Could you check a few things on this model? Use its own coordinates, in mm. A direction names the side the tool comes from. Coordinates: 2 decimals unless noted, no trailing zeros. Write each loop counter-clockwise with the first axis right and the second up, starting at its lowest first coordinate (ties: lowest second). Pieces come first, ordered by that corner, then holes. Notation, with made-up numbers: (20, -23) - (73, -23) arc R19 cw to (73, 2) - close; hole circle Ø3 at (-33, -13.5). An arc over 180 degrees is marked (long way). Answer as a JSON object with one key per item and string values. Group by question number.
1) Please list where these lines run through material, in increasing order: line 1 along Z through (x, y) = (49.5, 8.75) (3 decimals); line 2 along Y through (x, z) = (72, -6) (3 decimals); line 3 along X through (y, z) = (22.5, -28.5).
2) If we section it at B-B (x = 40): Write out the boundary of the cut face in (y, z) (3 decimals), plus the area to 3 significant figures.
3) If we section it at D-D (z = -9): Write out the boundary of the cut face in (x, y) (3 decimals), plus the area to 3 significant figures.
4) If we section it at C-C (y = 17.25): Write out the boundary of the cut face in (x, z) (3 decimals), plus the area to 3 significant figures.
5) We'd pull the mould along Z, two halves only. Please class faces 4 (the flat face through (0, 23, -25)), 5 (the flat face through (26, 24, -38.1)), 6 (the flat face through (50, 13, -50.8)), 7 (the flat face through (50, 22.225, -26)): released by +Z, released by -Z, zero draft, split by the parting line, or undercut.
6) If we section it at A-A (z = -27): Write out the boundary of the cut face in (x, y) (3 decimals).
7) On a 3-axis mill with a long thin cutter (end or side, diameter ignored), from which of +Z, -Z, +X, -X, +Y, -Y can I reach the whole of each face in a straight line? I mean faces 1 (the flat face through (50, 13, 0)), 2 (the flat face through (25, 24, -12.7)), 3 (the flat face through (50, 3.175, -25)). Say none if no direction works.
Autodesk Fusion 360 part; units mm, degrees
sketch "Sketch1" plane through (0, 0, 0) normal (1, 0, 0) x (0, 0, -1)
  line L0 (0, 0) -> (50.8, 0)
  line L1 (50.8, 0) -> (50.8, 25.4)
  line L2 (50.8, 25.4) -> (0, 25.4)
  line L3 (0, 25.4) -> (0, 0)
  line L4 (3.175, 3.175) -> (47.625, 3.175)
  line L5 (47.625, 3.175) -> (47.625, 22.225)
  line L6 (47.625, 22.225) -> (3.175, 22.225)
  line L7 (3.175, 22.225) -> (3.175, 3.175)
  dimension "d1" = 50.8
  dimension "d2" = 25.4
  dimension "d3" = -3.175
extrude "Extrude1" add sketch "Sketch1" along normal blind 101.6
sketch "Sketch2" plane through (0, 25.4, 0) normal (0, 1, 0) x (-1, 0, 0)
  line L0 (0, -50.8) -> (0, 0)
  line L1 (0, 0) -> (-101.6, 0)
  line L2 (-101.6, 0) -> (-101.6, -50.8)
  line L3 (-101.6, -50.8) -> (0, -50.8)
  line L4 (-12.7, -12.7) -> (-38.1, -12.7)
  line L5 (-38.1, -12.7) -> (-38.1, -38.1)
  line L6 (-38.1, -38.1) -> (-12.7, -38.1)
  line L7 (-12.7, -38.1) -> (-12.7, -12.7)
  dimension "d6" = 25.4
  dimension "d7" = 25.4
  dimension "d8" = 12.7
  dimension "d11" = 12.7
extrude "Extrude2" cut sketch "Sketch2" against normal blind 3.175 contours L4 L5 L6 L7
Here are the results:
{
 "1": {"line 1": "z = -50.8 to -47.625, -3.175 to 0", "line 2": "y = 0 to 3.175, 22.225 to 25.4", "line 3": "x = 0 to 12.7, 38.1 to 101.6"},
 "2": {"outline": "(0, -50.8) - (25.4, -50.8) - (25.4, 0) - (0, 0) - close; hole (3.175, -47.625) - (22.225, -47.625) - (22.225, -3.175) - (3.175, -3.175) - close", "area": "444 mm²"},
 "3": {"outline": "(0, 0) - (101.6, 0) - (101.6, 3.175) - (0, 3.175) - close; (0, 22.225) - (101.6, 22.225) - (101.6, 25.4) - (0, 25.4) - close", "area": "645 mm²"},
 "4": {"outline": "(0, -50.8) - (101.6, -50.8) - (101.6, -47.625) - (0, -47.625) - close; (0, -3.175) - (101.6, -3.175) - (101.6, 0) - (0, 0) - close", "area": "645 mm²"},
 "5": {"face 4": "zero draft", "face 5": "undercut", "face 6": "released by -Z", "face 7": "undercut"},
 "6": {"outline": "(0, 0) - (101.6, 0) - (101.6, 3.175) - (0, 3.175) - close; (0, 22.225) - (12.7, 22.225) - (12.7, 25.4) - (0, 25.4) - close; (38.1, 22.225) - (101.6, 22.225) - (101.6, 25.4) - (38.1, 25.4) - close"},
 "7": {"face 1": "+Z, +X, -X, +Y, -Y", "face 2": "+Y", "face 3": "+X, -X"}
}
